Verification items for the finished model (mm, model axes). Face numbers are marked on the shaded views. Give positions to 0.01 mm unless a question says otherwise; leave off trailing zeros. Order: outer loops, then holes, each group sorted by start corner. A loop starts at its lowest first (then second) coordinate and runs counter-clockwise, first axis right, second up.
from build123d import *

# Parameters (mm, degrees)
F1_DEPTH = 25
F3_D     = 4
F4_DEPTH = 25


with BuildPart() as f1:
    # F0 (on Front) → F1 (new body)
    with BuildSketch(Plane.XZ):
        Polygon((0, 0.2), (0, 0), (36, 0), (36, 5), align=None)
    extrude(amount=F1_DEPTH)

    # F3 (through all)
    with Locations(Plane(origin=(0, 0, 0), x_dir=(1, 0, 0), z_dir=(0, 0, -1))):
        with Locations((30.147626, 12.554323)):
            Hole(F3_D / 2)

    # F2 (on face) → F4 (cut)
    with BuildSketch(Plane(origin=(0, 0, 0), x_dir=(1, 0, 0), z_dir=(0, 0, -1))):
        with BuildLine():
            ThreePointArc((30.147626, 10.054323), (27.647626, 12.554323), (30.147626, 15.054323))
            Line((30.147626, 15.054323), (0, 15.054323))
            Line((0, 15.054323), (0, 10.054323))
            Line((0, 10.054323), (30.147626, 10.054323))
        make_face()
        with BuildLine():
            ThreePointArc((30.147626, 10.054323), (31.915393, 10.786556), (32.647626, 12.554323))
            ThreePointArc((32.647626, 12.554323), (31.915393, 14.32209), (30.147626, 15.054323))
            ThreePointArc((30.147626, 15.054323), (27.647626, 12.554323), (30.147626, 10.054323))
        make_face()
    extrude(amount=-F4_DEPTH, mode=Mode.SUBTRACT)


solid = f1.part
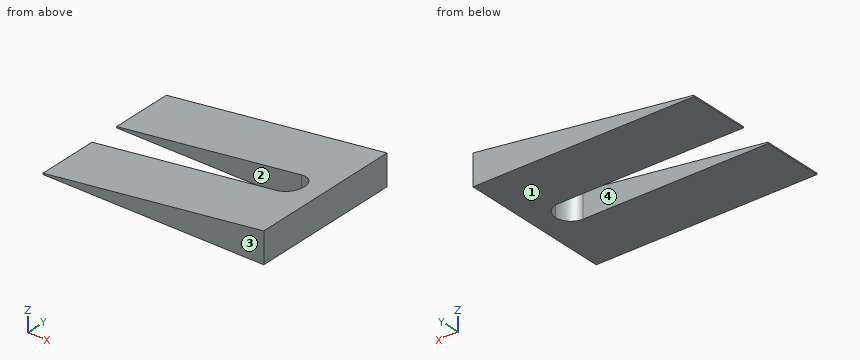
(1) Release check for a two-part mould opening along Y. For the marked faces 1, 2, 3 and 4 record: pulls with the +Y half, pulls with the -Y half, needs draft (parallel to the pull), parting line crosses it, or undercut.
Solved:
face 1: needs draft
face 2: undercut
face 3: pulls with the -Y half
face 4: undercut
(2) Section check D-D, the plane y = -5. Enter the section's corners in (x, z), then the cut area to 3 significant figures.
Solved:
outline: (0, 0) - (36, 0) - (36, 5) - (0, 0.2) - close
area: 93.6 mm2
(3) Section check C-C, the plane x = 3. Enter the section's corners in (y, z).
Solved:
outline: (-25, 0) - (-15.05, 0) - (-15.05, 0.6) - (-25, 0.6) - close; (-10.05, 0) - (0, 0) - (0, 0.6) - (-10.05, 0.6) - close
(4) Section check B-B, the plane z = 2.4. Enter the section's corners in (x, y).
Solved:
outline: (16.5, -25) - (36, -25) - (36, 0) - (16.5, 0) - (16.5, -10.05) - (30.15, -10.05) arc R2.5 cw to (30.15, -15.05) - (16.5, -15.05) - close
(5) Section check A-A, the plane x = 18. Enter the section's corners in (y, z).
Solved:
outline: (-25, 0) - (-15.05, 0) - (-15.05, 2.6) - (-25, 2.6) - close; (-10.05, 0) - (0, 0) - (0, 2.6) - (-10.05, 2.6) - close
(6) Scan lines: line 1 (Y direction, x = 19, z = 0.3); line 2 (Y direction, x = 31.5, z = 0.5); line 3 (Z direction, x = 30, y = -15.25). Record each from-to range of solid material in increasing order.
Solved:
line 1: y = -25 to -15.05, -10.05 to 0
line 2: y = -25 to -14.66, -10.45 to 0
line 3: z = 0 to 4.2
